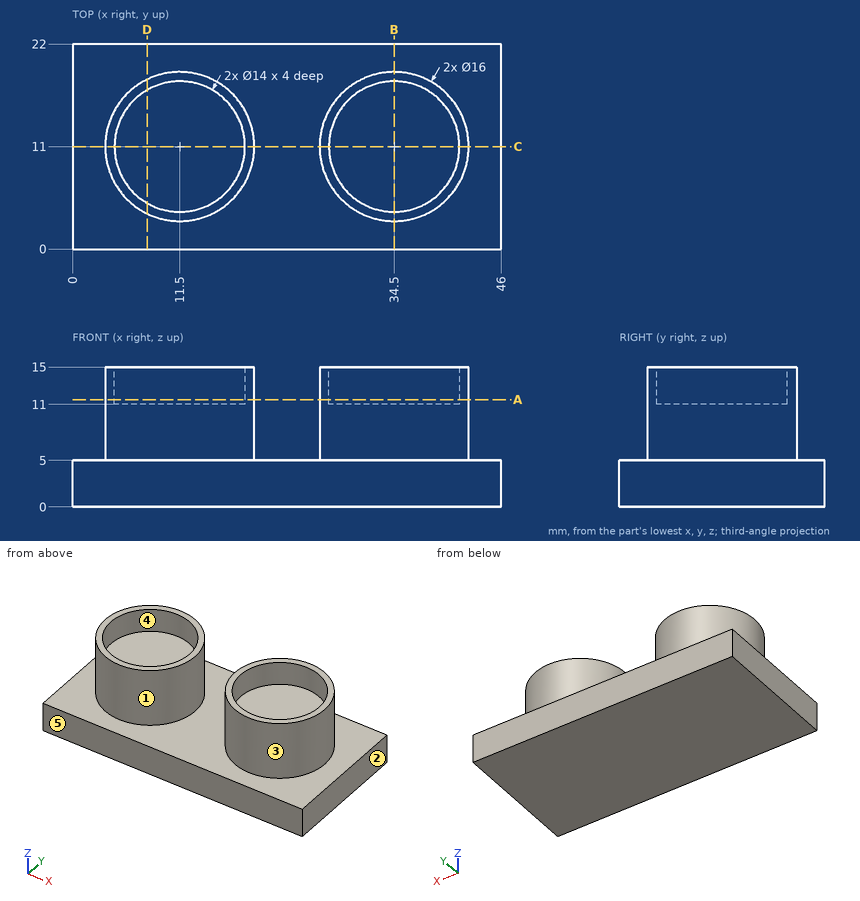
Here's the drawing with two shaded views (mm, measured from the low corner). I have some questions. A direction names the side the tool comes from. Coordinates: 2 decimals unless noted, no trailing zeros. Write each loop counter-clockwise with the first axis right and the second up, starting at its lowest first coordinate (ties: lowest second). Pieces come first, ordered by that corner, then holes. Notation, with made-up numbers: M 83.25,66 L 134.25,66 A10 ccw 134.25,83 Z; hole C -39,50.5 d2. An arc over 180 degrees is marked long. Answer as CSV lines item,"result". Start each with the question number.
1) For P1, Ø11, axis at x = 11.5, y = 15, coming from the +Z side; P2, Ø8, axis at y = 10, z = 13.5, coming from the -X side; P3, Ø1, axis at y = 17, z = 11, coming from the +X side; P4, Ø3, axis at x = 25, y = 16, coming from the +Z side, each with a flat end and sliding along its axis, tell me the tip position at first contact or that it passes through.
2) I want a section at D-D, the plane x = 8. Please give me the cut outline in (y, z).
3) For the marked faces 1 and 2, which set-ups out of +Z, -Z, +X, -X, +Y, -Y let a thin tool reach every point of the face, with its end or its side?
4) I want a section at A-A, the plane z = 11.5. Please give me the cut outline in (x, y), and give its area (3 significant figures).
5) I want a section at B-B, the plane x = 34.5. Please give me the cut outline in (y, z).
6) Please list where these lines run through material, in increasing order: line 1 (Y direction, x = 11.5, z = 13.1); line 2 (X direction, y = 6.5, z = 13); line 3 (X direction, y = 13.75, z = 14). Write a range as from..to.
7) I want a section at C-C, the plane y = 11. Please give me the cut outline in (x, z), and give its area (3 significant figures).
8) We'd pull the mould along Y, two halves only. Please class the marked faces 3, 4 and 5: +Y half, -Y half, draft (parallel to the pull), parting line (faces both ways), or undercut.
Data:
1,P1,"stops at z = 15"
1,P2,"stops at x = 3.5"
1,P3,"stops at x = 40.31"
1,P4,"stops at z = 5"
2,outline,"M 0,0 L 22,0 L 22,5 L 18.19,5 L 18.19,15 L 17.06,15 L 17.06,11 L 4.94,11 L 4.94,15 L 3.81,15 L 3.81,5 L 0,5 Z"
3,face 1,"+Z"
3,face 2,"+Z, -Z, +X, +Y, -Y"
4,outline,"C 11.5,11 d16; C 34.5,11 d16; hole C 11.5,11 d14; hole C 34.5,11 d14"
4,area,"94.2 mm^2"
5,outline,"M 0,0 L 22,0 L 22,5 L 19,5 L 19,15 L 18,15 L 18,11 L 4,11 L 4,15 L 3,15 L 3,5 L 0,5 Z"
6,line 1,"y = 3..4, 18..19"
6,line 2,"x = 4.89..6.14, 16.86..18.11, 27.89..29.14, 39.86..41.11"
6,line 3,"x = 3.99..5.06, 17.94..19.01, 26.99..28.06, 40.94..42.01"
7,outline,"M 0,0 L 46,0 L 46,5 L 42.5,5 L 42.5,15 L 41.5,15 L 41.5,11 L 27.5,11 L 27.5,15 L 26.5,15 L 26.5,5 L 19.5,5 L 19.5,15 L 18.5,15 L 18.5,11 L 4.5,11 L 4.5,15 L 3.5,15 L 3.5,5 L 0,5 Z"
7,area,"438 mm^2"
8,face 3,"parting line"
8,face 4,"undercut"
8,face 5,"-Y half"
